Autodesk Inventor part; units mm, degrees
ref_plane "YZ Plane" through (0, 0, 0) normal (1, 0, 0) x (0, 1, 0)
ref_plane "XZ Plane" through (0, 0, 0) normal (0, 1, 0) x (-1, 0, 0)
ref_plane "XY Plane" through (0, 0, 0) normal (0, 0, 1) x (1, 0, 0)
sketch "Эскиз1" plane through (0, 0, 0) normal (1, 0, 0) x (0, 1, 0)
  line L0 (0, 0) -> (8, 0)
  line L1 (8, 0) -> (8, -4)
  line L2 (8, -4) -> (22, -4)
  line L3 (22, -4) -> (22, 0)
  line L4 (22, 0) -> (38, 0)
  line L5 (38, 0) -> (38, -4)
  line L6 (38, -4) -> (52, -4)
  line L7 (52, -4) -> (52, 0)
  line L8 (52, 0) -> (60, 0)
  line L9 (60, 0) -> (60, 12)
  line L10 (60, 12) -> (64, 12)
  line L11 (64, 12) -> (64, 32)
  line L12 (64, 32) -> (60, 32)
  line L13 (60, 32) -> (60, 53)
  line L14 (60, 53) -> (64, 53)
  line L15 (64, 53) -> (64, 73)
  line L16 (64, 73) -> (60, 73)
  line L17 (60, 73) -> (60, 85)
  line L18 (-4, 65.2) -> (-4, 50)
  line L19 (-4, 50) -> (0, 50)
  line L20 (0, 50) -> (0, 33)
  line L21 (0, 33) -> (-4, 33)
  line L22 (-4, 33) -> (-4, 17)
  line L23 (-4, 17) -> (0, 17)
  line L24 (0, 17) -> (0, 0)
  line L25 (0, 61.2) -> (42.4, 61.2) construction
  line L26 (42.4, 61.2) -> (42.4, 18.8) construction
  line L27 (42.4, 18.8) -> (0, 18.8) construction
  line L28 (0, 18.8) -> (0, 61.2) construction
  line L29 (42.4, 61.2) -> (0, 18.8) construction
  line L30 (0, 61.2) -> (42.4, 18.8) construction
  circle A0 centre (21.2, 40) radius 11
  circle A1 centre (36.7, 55.5) radius 1.5
  circle A2 centre (36.7, 24.5) radius 1.5
  circle A3 centre (5.7, 24.5) radius 1.5
  circle A4 centre (5.7, 55.5) radius 1.5
  line L31 (-4, 65.2) -> (14, 85)
  line L32 (27, 85) -> (27, 81)
  line L33 (27, 81) -> (47, 81)
  line L34 (47, 81) -> (47, 85)
  line L35 (47, 85) -> (60, 85)
  line L36 (15, 14.8) -> (45, 14.8)
  line L37 (45, 14.8) -> (45, 18.8)
  line L38 (45, 18.8) -> (15, 18.8)
  line L39 (15, 18.8) -> (15, 14.8)
  line L40 (15, 61.2) -> (45, 61.2)
  line L41 (45, 61.2) -> (45, 65.2)
  line L42 (45, 65.2) -> (15, 65.2)
  line L43 (15, 65.2) -> (15, 61.2)
  line L44 (14, 85) -> (14, 75)
  line L45 (14, 75) -> (18, 75)
  line L46 (18, 75) -> (18, 85)
  line L47 (18, 85) -> (27, 85)
  point P0 (21.2, 40)
  point P1 (30, 14.8)
  point P2 (30, 0)
  dimension "d0" = 4
  dimension "d1" = 8
  dimension "d2" = 14
  dimension "d3" = 16
  dimension "d4" = 14
  dimension "d5" = 8
  dimension "d6" = 17
  dimension "d7" = 16
  dimension "d8" = 17
  dimension "d9" = 15.2
  dimension "d11" = 12
  dimension "d12" = 20
  dimension "d13" = 20
  dimension "d16" = 21
  dimension "d22" = 42.4
  dimension "d23" = 31
  dimension "d24" = 40
  dimension "d25" = 22
  dimension "d26" = 3
  dimension "d31" = 85
  dimension "d32" = 12
  dimension "d33" = 20
  dimension "d36" = 30
  dimension "d37" = 10
  dimension "d38" = 13
  dimension "d40" = 13
extrude "Выдавливание1" add sketch "Эскиз1" along normal blind 4
sketch "Эскиз4" plane through (4, 0, 0) normal (1, 0, 0) x (0, 0, -1)
  line L0 (0, 0) -> (0, 8)
  line L1 (-14.8, 45) -> (-14.8, 15)
  line L2 (-17, 0) -> (0, 0)
  line L3 (0, 60) -> (-12, 60)
  line L4 (-73, 60) -> (-85, 60)
  line L5 (-65.2, 15) -> (-65.2, 45)
  point P0 (-9.8, 14)
  point P1 (-9.8, 46)
  point P2 (-71.2, 51)
  point P3 (-71.2, 27)
  dimension "d51" = 5
  dimension "d52" = 14
  dimension "d53" = 14
  dimension "d54" = 9
  dimension "d55" = 33
  dimension "d56" = 6
hole "Отверстие1" at (4, 14, 9.8) at (4, 46, 9.8) at (4, 51, 71.2) at (4, 27, 71.2) direction (-1, 0, 0) diameter 2.8 end through all
properties part number "stepperMount" material "Дерево (береза)"
Geometry check sheet. Reference: the model listing, model coordinates, mm. A direction names the side the tool comes from. Round coordinates to 2 decimals unless told otherwise and drop trailing zeros. Write each loop counter-clockwise with the first axis right and the second up, starting at its lowest first coordinate (ties: lowest second). Pieces come first, ordered by that corner, then holes.
Item 1: Mould release check, pull along Y, two halves, no side actions. Record for faces 4 (the face through (2, 15, 17)), 5 (the face through (2, 4, 0)), 6 (the face through (2, -4, 25)): +Y half, -Y half, draft (parallel to the pull), parting line (faces both ways), or undercut.
Determined:
face 4: undercut
face 5: draft
face 6: -Y half
Item 2: Go/stop test with flat-tipped pins: pin 1 Ø1.2 at (x, z) = (2.5, 82) entering from +Y; pin 2 Ø1.2 at (x, y) = (1.5, 15.5) entering from +Z; pin 3 Ø2 at (x, y) = (2, 32.5) entering from -Z. Record where each tip stops, or that it passes through.
Determined:
pin 1: stops at y = 60
pin 2: stops at z = 75
pin 3: stops at z = 0
Item 3: Section check C-C (z = 79.5). Record the boundary of the cut face in (x, y), plus the area to 3 significant figures.
Determined:
outline: (0, 9) - (4, 9) - (4, 14) - (0, 14) - close; (0, 18) - (4, 18) - (4, 60) - (0, 60) - close
area: 188 mm2
Item 4: Material ranges on line 1 along Z through (x, y) = (2.8, 36.7); line 2 along Z through (x, y) = (0.2, 30.5); line 3 along Z through (x, y) = (0.55, 42.5), recorded low to high.
Determined:
line 1: z = 0 to 14.8, 18.8 to 23, 26 to 54, 57 to 61.2, 65.2 to 81
line 2: z = 0 to 14.8, 18.8 to 34.13, 45.87 to 61.2, 65.2 to 81
line 3: z = -4 to 14.8, 18.8 to 61.2, 65.2 to 81
Item 5: Section check B-B (y = 5.7). Record the boundary of the cut face in (x, z), plus the area to 3 significant figures.
Determined:
outline: (0, 0) - (4, 0) - (4, 23) - (0, 23) - close; (0, 26) - (4, 26) - (4, 54) - (0, 54) - close; (0, 57) - (4, 57) - (4, 75.87) - (0, 75.87) - close
area: 279 mm2
Item 6: Access from +Z, -Z, +X, -X, +Y, -Y to the whole of each face (thin tool, end or side, straight path). Record for faces 1 (the face through (2, 30, 18.8)), 2 (the face through (2, 8, -2)), 3 (the face through (2, 37, 81)).
Determined:
face 1: +X, -X
face 2: -Z, +X, -X, -Y
face 3: +Z, +X, -X
Item 7: Section check A-A (z = 24.5). Record the boundary of the cut face in (x, y), plus the area to 3 significant figures.
Determined:
outline: (0, -4) - (4, -4) - (4, 4.2) - (0, 4.2) - close; (0, 7.2) - (4, 7.2) - (4, 35.2) - (0, 35.2) - close; (0, 38.2) - (4, 38.2) - (4, 64) - (0, 64) - close
area: 248 mm2
Item 8: Section check D-D (y = 46). Record the boundary of the cut face in (x, z), plus the area to 3 significant figures.
Determined:
outline: (0, -4) - (4, -4) - (4, 8.4) - (0, 8.4) - close; (0, 11.2) - (4, 11.2) - (4, 81) - (0, 81) - close
area: 329 mm2
